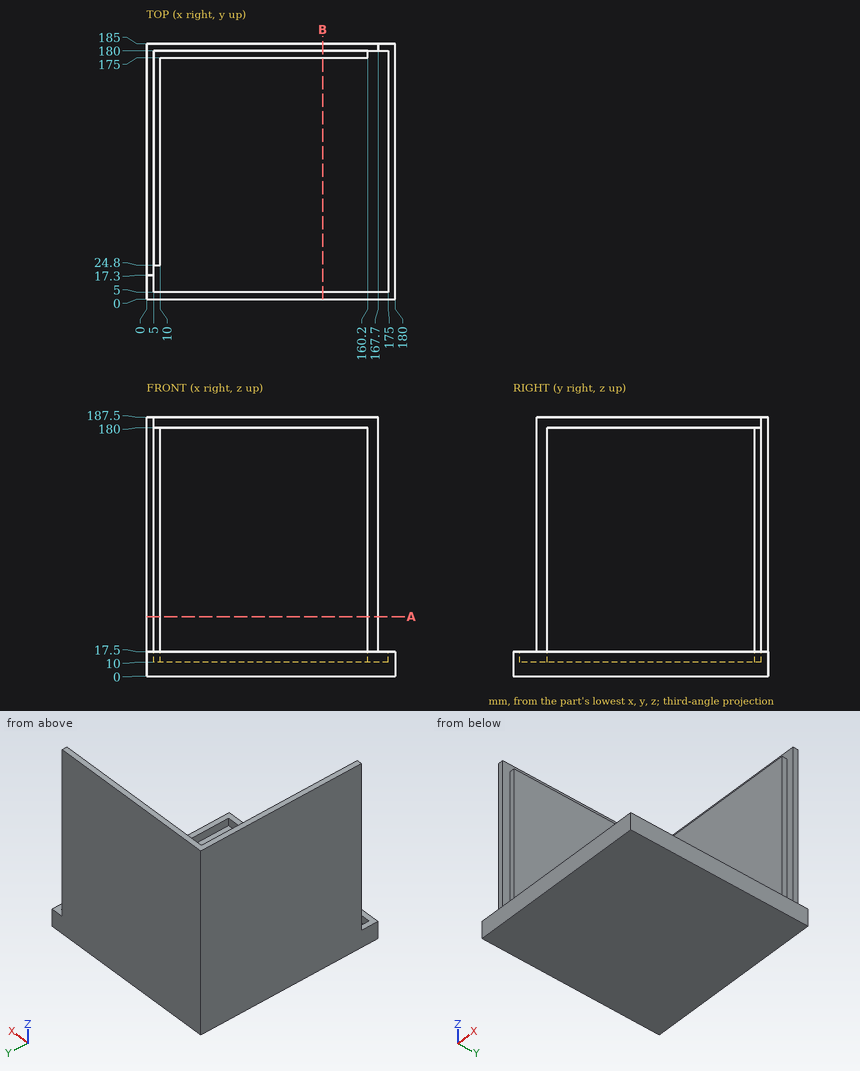
Input: dimensioned drawing with shaded views. Units: mm. Origin: part minimum x, y, z. Coordinates: 2 decimals unless noted, no trailing zeros. Order: outer loops, then holes, each group sorted by start corner. A loop starts at its lowest first (then second) coordinate and runs counter-clockwise, first axis right, second up. Notation, with made-up numbers: (55.5, 26.5) - (60.5, 26.5) arc R26 cw to (60.5, 63.5) - close; hole circle Ø9 at (2.25, 33). An arc over 180 degrees is marked (long way). One line per item, written item: value.
1) Cut plane A-A on z = 43. Output: boundary loops of the cut face in (x, y), plus the area to 3 significant figures.
Computed values:
outline: (0, 17.3) - (5, 17.3) - (5, 24.8) - (10, 24.8) - (10, 175) - (160.2, 175) - (160.2, 180) - (167.7, 180) - (167.7, 185) - (0, 185) - close
area: 3,180 mm^2
2) Ray query, line 1 (Y direction, x = 34, z = 13.5); line 2 (Y direction, x = 60, z = 110.5); line 3 (Z direction, x = 19, y = 67). Return the intervals inside material, ascending. Write a range as [from, to].
Computed values:
line 1: y = [0, 5], [175, 185]
line 2: y = [175, 185]
line 3: z = [0, 10]
3) Contact query for flat-ended pins moving along their axis: pin 1 (1 mm diameter, centred on x = 22.5, z = 43, fed in from -Y); pin 2 (1 mm diameter, centred on y = 75.5, z = 103.5, fed in from +X); pin 3 (1.5 mm diameter, centred on y = 177.5, z = 128.5, fed in from +X). Output: stop coordinate, or through.
Computed values:
pin 1: stops at y = 175
pin 2: stops at x = 10
pin 3: stops at x = 160.2
4) Cut plane B-B on x = 127.5. Output: boundary loops of the cut face in (y, z), plus the area to 4 significant figures.
Computed values:
outline: (0, 0) - (185, 0) - (185, 187.5) - (180, 187.5) - (180, 180) - (175, 180) - (175, 10) - (5, 10) - (5, 17.5) - (0, 17.5) - close
area: 3,625 mm^2
